```python
from build123d import *

# Parameters (mm, degrees)
SKETCH2_R           = 4
BOSS_EXTRUDE1_DEPTH = 4.33
SKETCH3_R           = 1
CUT_EXTRUDE1_DEPTH  = 5
SKETCH4_R           = 1
CUT_EXTRUDE2_DEPTH  = 5
SKETCH5_R           = 1
CUT_EXTRUDE3_DEPTH  = 5
SKETCH6_R           = 1
CUT_EXTRUDE4_DEPTH  = 5


with BuildPart() as part:
    # Sketch2 → Boss-Extrude1 (new body)
    with BuildSketch(Plane(origin=(0, 0, 0), x_dir=(1, 0, 0), z_dir=(0, 1, 0))):
        Polygon((0, 0), (12, 0), (12, 12.85), (23.5, 12.85), (23.5, 24.85), (12, 24.85), (12, 38.72), (0, 38.72), (0, 24.85), (-11.5, 24.85), (-11.5, 12.85), (0, 12.85), align=None)
        with Locations((6, 18.85)):
            Circle(SKETCH2_R, mode=Mode.SUBTRACT)
    extrude(amount=BOSS_EXTRUDE1_DEPTH)

    # Sketch3 → Cut-Extrude1 (cut)
    with BuildSketch(Plane.XY):
        with Locations((3, 2.165)):
            Circle(SKETCH3_R)
        with Locations((9, 2.165)):
            Circle(SKETCH3_R)
    extrude(amount=-CUT_EXTRUDE1_DEPTH, mode=Mode.SUBTRACT)

    # Sketch4 → Cut-Extrude2 (cut)
    with BuildSketch(Plane.ZY.offset(11.5)):
        with Locations((-21.85, 2.165)):
            Circle(SKETCH4_R)
        with Locations((-15.85, 2.165)):
            Circle(SKETCH4_R)
    extrude(amount=-CUT_EXTRUDE2_DEPTH, mode=Mode.SUBTRACT)

    # Sketch5 → Cut-Extrude3 (cut)
    with BuildSketch(Plane(origin=(0, 0, -38.72), x_dir=(-1, 0, 0), z_dir=(0, 0, -1))):
        with Locations((-9, 2.165)):
            Circle(SKETCH5_R)
        with Locations((-3, 2.165)):
            Circle(SKETCH5_R)
    extrude(amount=-CUT_EXTRUDE3_DEPTH, mode=Mode.SUBTRACT)

    # Sketch6 → Cut-Extrude4 (cut)
    with BuildSketch(Plane(origin=(23.5, 0, 0), x_dir=(0, 0, -1), z_dir=(1, 0, 0))):
        with Locations((15.85, 2.165)):
            Circle(SKETCH6_R)
        with Locations((21.85, 2.165)):
            Circle(SKETCH6_R)
    extrude(amount=-CUT_EXTRUDE4_DEPTH, mode=Mode.SUBTRACT)


solid = part.part
```
Source: CAD feature listing. Evaluate the final solid. Frame: model axes, mm. A direction names the side the tool comes from. Coordinates: 2 decimals unless noted, no trailing zeros. Loops run counter-clockwise (first coordinate to the right, second up) from the corner with the lowest first, then second, coordinate; pieces in that order, holes last. Notation, with made-up numbers: M 46,-1.5 L 78,-1.5 A29 cw 78,24.5 Z; hole C -5,30.25 d7. An arc over 180 degrees is marked long. Put each result on its own line as item: value. Start each with the question number.
1) Pull-direction query (Z, two-part tool) for faces 1 (the face through (-6, 2, -24.85)), 2 (the face through (21.035, 2.465, -16.804)), 3 (the face through (3.13, 3.156, -36.255)); classes: pulls with the +Z half, pulls with the -Z half, needs draft (parallel to the pull), parting line crosses it, or undercut.
2) Cut plane A-A on z = -18.85. Return the cut outline in (x, y).
3) Ray query, L1, parallel to Y at x = -9.25, z = -21.85 (3 decimals); L2, parallel to Z at x = 6, y = 3.3; L3, parallel to X at y = 2.65, z = -3. Return the intervals inside material, ascending. Write a range as from..to.
4) Cut plane B-B on x = 3.5. Return the cut outline in (y, z).
5) Cut plane D-D on x = 19.5. Return the cut outline in (y, z) (3 decimals).
6) Reachability of faces 4 (the face through (12, 2, -6)), 5 (the face through (18.5, 2, -22)), 6 (the face through (0, 2, -32)), 7 (the face through (-9, 3, -15.3)), 8 (the face through (8.26, 2.84, -2.46)) from +Z, -Z, +X, -X, +Y, -Y: full face, straight path, thin tool, end or side. Return the list, or none.
7) Cut plane C-C on y = 3.7. Return the cut outline in (x, z), then the cut area to 3 significant figures.
8) Contact query for flat-ended pins moving along their axis: pin 1 Ø1.6 at (x, y) = (9, 2.165) entering from -Z; pin 2 Ø2 at (y, z) = (2, -6) entering from -X; pin 3 Ø2 at (y, z) = (2.5, -30) entering from +X. Output: stop coordinate, or through.
The answers:
1. face 1: pulls with the -Z half
1. face 2: undercut
1. face 3: needs draft
2. outline: M -11.5,0 L 2,0 L 2,4.33 L -11.5,4.33 Z; M 10,0 L 23.5,0 L 23.5,4.33 L 10,4.33 Z
3. L1: y = 0..1.165, 3.165..4.33
3. L2: z = -38.72..-22.85, -14.85..0
3. L3: x = 0..2.13, 3.87..8.13, 9.87..12
4. outline: M 0,-38.72 L 1.3,-38.72 L 1.3,-33.72 L 3.03,-33.72 L 3.03,-38.72 L 4.33,-38.72 L 4.33,-21.97 L 0,-21.97 Z; M 0,-15.73 L 4.33,-15.73 L 4.33,0 L 3.03,0 L 3.03,-5 L 1.3,-5 L 1.3,0 L 0,0 Z
5. outline: M 0,-24.85 L 4.33,-24.85 L 4.33,-12.85 L 0,-12.85 Z; hole C 2.165,-21.85 d2; hole C 2.165,-15.85 d2
6. face 4: +Z, +X, +Y, -Y
6. face 5: +X
6. face 6: -Z, -X, +Y, -Y
6. face 7: -X
6. face 8: +Z
7. outline: M -11.5,-24.85 L 0,-24.85 L 0,-38.72 L 12,-38.72 L 12,-24.85 L 23.5,-24.85 L 23.5,-12.85 L 12,-12.85 L 12,0 L 0,0 L 0,-12.85 L -11.5,-12.85 Z; hole C 6,-18.85 d8
7. area: 690 mm²
8. pin 1: stops at z = -33.72
8. pin 2: stops at x = 0
8. pin 3: stops at x = 12
